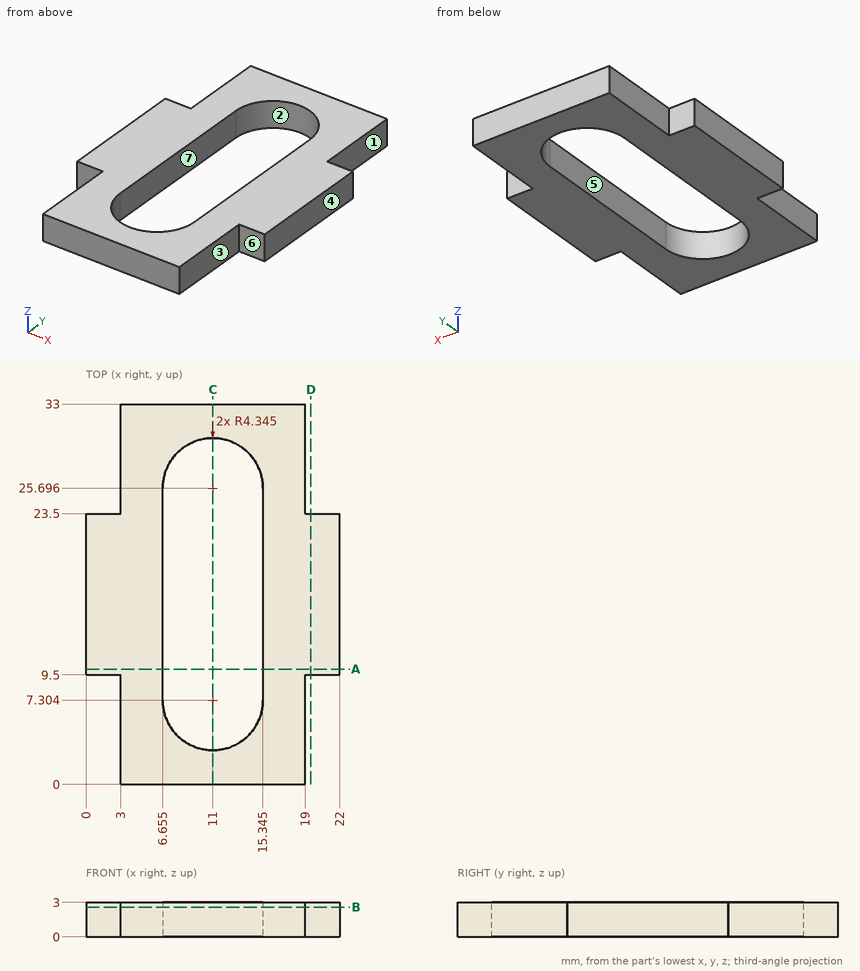
The drawing under review shows one solid part. Ordinate dimensions are in mm from its lowest x, y, z. A direction names the side the tool comes from. Round coordinates to 2 decimals unless told otherwise and drop trailing zeros. Order: outer loops, then holes, each group sorted by start corner. A loop starts at its lowest first (then second) coordinate and runs counter-clockwise, first axis right, second up. Notation, with made-up numbers: (15.5, 73.25) -> (25.5, 73.25) arc R22 ccw to (25.5, 110.25) -> close; hole circle Ø11 at (78.25, 22). An arc over 180 degrees is marked (long way). Use a Markdown table: item, result.
Item 1: For line 1 along X through (y, z) = (20, 0.25) (1 decimal); line 2 along X through (y, z) = (8, 1.7) (1 decimal); line 3 along Y through (x, z) = (14.25, 1.3), list the stretches that pass through material, from the lowest coordinate up. Write a range as [from, to].
Resolved:
| item | result |
|---|---|
| line 1 | x = [0, 6.7], [15.3, 22] |
| line 2 | x = [3, 6.7], [15.3, 19] |
| line 3 | y = [0, 4.42], [28.58, 33] |
Item 2: Take a section at B-B (z = 2.6). State the section outline as (x, y) points (1 decimal), plus the area to 3 significant figures.
Resolved:
| item | result |
|---|---|
| outline | (0, 9.5) -> (3, 9.5) -> (3, 0) -> (19, 0) -> (19, 9.5) -> (22, 9.5) -> (22, 23.5) -> (19, 23.5) -> (19, 33) -> (3, 33) -> (3, 23.5) -> (0, 23.5) -> close; hole (6.7, 7.3) arc R4.3 ccw to (15.3, 7.3) -> (15.3, 25.7) arc R4.3 ccw to (6.7, 25.7) -> close |
| area | 393 mm² |
Item 3: Take a section at C-C (x = 11). State the section outline as (y, z) points.
Resolved:
| item | result |
|---|---|
| outline | (0, 0) -> (2.96, 0) -> (2.96, 3) -> (0, 3) -> close; (30.04, 0) -> (33, 0) -> (33, 3) -> (30.04, 3) -> close |
Item 4: Take a section at D-D (x = 19.5). State the section outline as (y, z) points, plus the area to 3 significant figures.
Resolved:
| item | result |
|---|---|
| outline | (9.5, 0) -> (23.5, 0) -> (23.5, 3) -> (9.5, 3) -> close |
| area | 42.0 mm² |
Item 5: Draft analysis for pull direction X (two halves, no side actions). For the marked faces 4, 5, 6 and 7, state which applies: +X half, -X half, draft (parallel to the pull), parting line (faces both ways), or undercut.
Resolved:
| item | result |
|---|---|
| face 4 | +X half |
| face 5 | undercut |
| face 6 | draft |
| face 7 | undercut |
Item 6: Take a section at A-A (y = 10). State the section outline as (x, z) points (1 decimal).
Resolved:
| item | result |
|---|---|
| outline | (0, 0) -> (6.7, 0) -> (6.7, 3) -> (0, 3) -> close; (15.3, 0) -> (22, 0) -> (22, 3) -> (15.3, 3) -> close |
Item 7: For pin 1 (1.5 mm diameter, centred on x = 1, z = 1, fed in from -Y); pin 2 (0.9 mm diameter, centred on y = 30.5, z = 1.5, fed in from +X); pin 3 (10 mm diameter, centred on x = 9, y = 24, fed in from +Z); pin 4 (1.5 mm diameter, centred on x = 21, z = 1.5, fed in from +Y), all flat-tipped, find the tip position at first contact; note any pin that passes through.
Resolved:
| item | result |
|---|---|
| pin 1 | stops at y = 9.5 |
| pin 2 | stops at x = 19 |
| pin 3 | stops at z = 3 |
| pin 4 | stops at y = 23.5 |
Item 8: Machinability: for the marked faces 1, 2 and 3, which of the approach directions +Z, -Z, +X, -X, +Y, -Y give a long, thin tool a straight path to every point of the face, cutting with its end or side? Answer none if there is none.
Resolved:
| item | result |
|---|---|
| face 1 | +Z, -Z, +X, +Y |
| face 2 | +Z, -Z |
| face 3 | +Z, -Z, +X, -Y |
